Check sheet for the modelled part. Datum: model origin and axes. Units: mm. A direction names the side the tool comes from. Coordinates: 2 decimals unless noted, no trailing zeros. Order: outer loops, then holes, each group sorted by start corner. A loop starts at its lowest first (then second) coordinate and runs counter-clockwise, first axis right, second up.
1. Draft check along X on faces 3 (the flat face through (1.4, 0.25, 1.4)), 4 (the flat face through (3, 0.5, 2)), 5 (the cylindrical face through (-0.83, -0.01, -3.76)). Enter one of: released by +X, released by -X, zero draft, split by the parting line, or undercut.
2. Cross-section at B-B (x = 0). Enter the section's corners in (y, z), then the cut area to 3 significant figures.
3. Cross-section at C-C (y = 0.35). Enter the section's corners in (x, z).
4. Set-up check for faces 1 (the flat face through (1.4, -0.25, -1.4)), 2 (the flat face through (3, -0.5, 2)): record each of +Z, -Z, +X, -X, +Y, -Y from which the full face is reachable in a straight line by a thin tool's end or side.
5. Thickness scan on line 1 (Z direction, x = 0, y = 0.45); line 2 (X direction, y = 0.2, z = 1); line 3 (Y direction, x = -1, z = -2.5). Record the ranges inside material, lowest first.
6. Cross-section at A-A (z = 0). Enter the section's corners in (x, y), then the cut area to 3 significant figures.
7. Gauge pin test, flat ends, axial feed: pin 1 Ø1 at (x, z) = (1, 1.5) entering from +Y; pin 2 Ø1 at (x, z) = (0.5, -1) entering from -Y; pin 3 Ø0.6 at (x, y) = (-2, 0) entering from -Z. Record the tip position at first contact, or that the pin passes through.
```python
from build123d import *

# Parameters (mm, degrees)
BASE_W             = 2.5
BASE_H             = 1
SKETCH1_R          = 4
SKETCH1_R_2        = 3.85
CUT_EXTRUDE1_DEPTH = 10
SKETCH6_R          = 3.25
CUT_EXTRUDE5_DEPTH = 0.25
CUT_EXTRUDE6_START = -0.25
SKETCH7_R          = 3.25
CUT_EXTRUDE6_DEPTH = 0.25
SKETCH4_W          = 6
SKETCH4_H          = 1.5
SKETCH4_W_2        = 1.5
SKETCH4_H_2        = 6
CUT_EXTRUDE4_DEPTH = 10


with BuildPart() as part:
    # base → Revolution (revolve)
    with BuildSketch(Plane.XY):
        with Locations((2.75, 0)):
            Rectangle(BASE_W, BASE_H)
    revolve(axis=Axis((0, -0.5, 0), (0, 1, 0)))

    # Sketch1 → Cut-Extrude1 (cut)
    with BuildSketch(Plane(origin=(0, -0.5, 0), x_dir=(-1, 0, 0), z_dir=(0, -1, 0))):
        Circle(SKETCH1_R)
        with Locations(Location((0, 0, 0), (0, 0, 180))):
            Circle(SKETCH1_R_2, mode=Mode.SUBTRACT)
    extrude(amount=-CUT_EXTRUDE1_DEPTH, mode=Mode.SUBTRACT)

    # Sketch6 → Cut-Extrude5 (cut)
    with BuildSketch(Plane(origin=(0, -0.5, 0), x_dir=(-1, 0, 0), z_dir=(0, -1, 0))):
        with Locations(Location((0, 0, 0), (0, 0, 180))):
            Circle(SKETCH6_R)
    extrude(amount=-CUT_EXTRUDE5_DEPTH, mode=Mode.SUBTRACT)

    # Sketch7 → Cut-Extrude6 (cut)
    with BuildSketch(Plane(origin=(0, 0.5, 0), x_dir=(1, 0, 0), z_dir=(0, 1, 0)).offset(CUT_EXTRUDE6_START)):
        Circle(SKETCH7_R)
    extrude(amount=CUT_EXTRUDE6_DEPTH, mode=Mode.SUBTRACT)

    # Sketch4 → Cut-Extrude4 (cut)
    with BuildSketch(Plane(origin=(0, -0.5, 0), x_dir=(-1, 0, 0), z_dir=(0, -1, 0))):
        Rectangle(SKETCH4_W, SKETCH4_H)
        Rectangle(SKETCH4_W_2, SKETCH4_H_2)
    extrude(amount=-CUT_EXTRUDE4_DEPTH, mode=Mode.SUBTRACT)


solid = part.part
```
Data:
1. face 3: undercut
1. face 4: zero draft
1. face 5: split by the parting line
2. outline: (-0.5, -3.85) - (0.5, -3.85) - (0.5, -3.25) - (0.25, -3.25) - (0.25, -3) - (-0.25, -3) - (-0.25, -3.25) - (-0.5, -3.25) - close; (-0.5, 3.25) - (-0.25, 3.25) - (-0.25, 3) - (0.25, 3) - (0.25, 3.25) - (0.5, 3.25) - (0.5, 3.85) - (-0.5, 3.85) - close
2. area: 1.45 mm2
3. outline: circle Ø7.7 at (0, 0); hole circle Ø6.5 at (0, 0)
4. face 1: -Y
4. face 2: +Z, -Z, +X, -X, -Y
5. line 1: z = -3.85 to -3.25, 3.25 to 3.85
5. line 2: x = -3.72 to -1.12, 1.12 to 3.72
5. line 3: y = -0.25 to 0.25
6. outline: (-3.85, -0.5) - (-3.25, -0.5) - (-3.25, -0.25) - (-3, -0.25) - (-3, 0.25) - (-3.25, 0.25) - (-3.25, 0.5) - (-3.85, 0.5) - close; (3, -0.25) - (3.25, -0.25) - (3.25, -0.5) - (3.85, -0.5) - (3.85, 0.5) - (3.25, 0.5) - (3.25, 0.25) - (3, 0.25) - close
6. area: 1.45 mm2
7. pin 1: stops at y = 0.25
7. pin 2: stops at y = -0.25
7. pin 3: stops at z = -3.45
